from build123d import *

# Parameters (mm, degrees)
SKETCH1_R           = 12.5
BOSS_EXTRUDE1_DEPTH = 25
SKETCH2_R           = 5
CUT_EXTRUDE1_DEPTH  = 20
SKETCH4_R           = 2
CUT_EXTRUDE2_DEPTH  = 20
SKETCH5_R           = 28.5
SKETCH5_R_2         = 2.6
BOSS_EXTRUDE2_DEPTH = 6
SKETCH6_R           = 9
BOSS_EXTRUDE3_DEPTH = 80.52
SKETCH7_R           = 8.5
BOSS_EXTRUDE4_DEPTH = 20.5
SKETCH8_R           = 10.9
BOSS_EXTRUDE5_DEPTH = 18


with BuildPart() as part:
    # Sketch1 → Boss-Extrude1 (new body)
    with BuildSketch(Plane.XY):
        Circle(SKETCH1_R)
    extrude(amount=BOSS_EXTRUDE1_DEPTH)

    # Sketch2 → Cut-Extrude1 (cut)
    with BuildSketch(Plane(origin=(0, 0, 0), x_dir=(-1, 0, 0), z_dir=(0, 0, -1))):
        Circle(SKETCH2_R)
    extrude(amount=-CUT_EXTRUDE1_DEPTH, mode=Mode.SUBTRACT)

    # Sketch4 → Cut-Extrude2 (cut)
    with BuildSketch(Plane(origin=(0, 0, 0), x_dir=(1, 0, 0), z_dir=(0, 1, 0))):
        with Locations(Location((0, -8, 0), (0, 0, 270))):
            Circle(SKETCH4_R)
    extrude(amount=-CUT_EXTRUDE2_DEPTH, mode=Mode.SUBTRACT)

    # Sketch5 → Boss-Extrude2 (add)
    with BuildSketch(Plane.XY.offset(25)):
        Circle(SKETCH5_R)
        with Locations((0, 23.75)):
            Circle(SKETCH5_R_2, mode=Mode.SUBTRACT)
        with Locations((20.56810334, 11.875)):
            Circle(SKETCH5_R_2, mode=Mode.SUBTRACT)
        with Locations((20.56810334, -11.875)):
            Circle(SKETCH5_R_2, mode=Mode.SUBTRACT)
        with Locations((0, -23.75)):
            Circle(SKETCH5_R_2, mode=Mode.SUBTRACT)
        with Locations((-20.56810334, -11.875)):
            Circle(SKETCH5_R_2, mode=Mode.SUBTRACT)
        with Locations((-20.56810334, 11.875)):
            Circle(SKETCH5_R_2, mode=Mode.SUBTRACT)
    extrude(amount=BOSS_EXTRUDE2_DEPTH)

    # Sketch6 → Boss-Extrude3 (add)
    with BuildSketch(Plane.XY.offset(31)):
        Circle(SKETCH6_R)
    extrude(amount=BOSS_EXTRUDE3_DEPTH)

    # Sketch7 → Boss-Extrude4 (add)
    with BuildSketch(Plane.XY.offset(111.52)):
        Circle(SKETCH7_R)
    extrude(amount=BOSS_EXTRUDE4_DEPTH)

    # Sketch8 → Boss-Extrude5 (add)
    with BuildSketch(Plane.XY.offset(31)):
        Circle(SKETCH8_R)
    extrude(amount=BOSS_EXTRUDE5_DEPTH)


solid = part.part
CAD build for the part. Positions are in the model's coordinates, mm. A direction names the side the tool comes from. Give positions to 0.01 mm unless a question says otherwise; leave off trailing zeros. Order: outer loops, then holes, each group sorted by start corner. A loop starts at its lowest first (then second) coordinate and runs counter-clockwise, first axis right, second up. Notation, with made-up numbers: (-4.5, 34) -> (18.5, 34) arc R24 ccw to (18.5, 45) -> close; hole circle Ø8 at (66, 36.5). An arc over 180 degrees is marked (long way). Return JSON: item names as keys, results as strings.
Q1. Saw through at D-D (z = 15.5). Write the cut outline in (x, y), then the cut area to 3 significant figures.
Working result:
{"outline": "circle Ø25 at (0, 0); hole circle Ø10 at (0, 0)", "area": "412 mm²"}
Q2. Drill centre lines: line 1 (Y direction, x = 0, z = 28); line 2 (Z direction, x = 0, y = -6.25); line 3 (Y direction, x = 18.5, z = 27). Where is each one in solid material? Low to high.
Working result:
{"line 1": "-28.5 to -26.35, -21.15 to 21.15, 26.35 to 28.5", "line 2": "0 to 6, 10 to 132.02", "line 3": "-21.68 to -13.45, -10.3 to 10.3, 13.45 to 21.68"}
Q3. Mould opens along X. For faces 1 (the face through (21.77, 9.57, 27.96)), 2 (the face through (-1.172, 8.923, 79.822)), 3 (the face through (-19.368, 9.568, 27.958)), 4 (the face through (-0.2, -5.4, 0)) say: pulls with the +X half, pulls with the -X half, needs draft (parallel to the pull), parting line crosses it, or undercut.
Working result:
{"face 1": "undercut", "face 2": "parting line crosses it", "face 3": "undercut", "face 4": "needs draft"}
Q4. Saw through at B-B (x = 20). Write the cut outline in (y, z), then the cut area to 3 significant figures.
Working result:
{"outline": "(-20.3, 25) -> (-14.41, 25) -> (-14.41, 31) -> (-20.3, 31) -> close; (-9.34, 25) -> (9.34, 25) -> (9.34, 31) -> (-9.34, 31) -> close; (14.41, 25) -> (20.3, 25) -> (20.3, 31) -> (14.41, 31) -> close", "area": "183 mm²"}
Q5. Which spindle directions (+Z, -Z, +X, -X, +Y, -Y) get a long thin tool onto all of the face, cutting with end or side? Do faces 5 (the face through (2, 9, 49)), 6 (the face through (0, 0, 132.02)), 7 (the face through (-0.338, 26.328, 27.958)), 8 (the face through (-0.766, -8.488, 9.847)), 9 (the face through (11.923, 3.755, 12.325)). Say none if no direction does.
Working result:
{"face 5": "+Z", "face 6": "+Z, +X, -X, +Y, -Y", "face 7": "+Z, -Z", "face 8": "-Y", "face 9": "-Z"}
Q6. Saw through at A-A (y = -23.75). Write the cut outline in (x, z).
Working result:
{"outline": "(-15.75, 25) -> (-2.6, 25) -> (-2.6, 31) -> (-15.75, 31) -> close; (2.6, 25) -> (15.75, 25) -> (15.75, 31) -> (2.6, 31) -> close"}
Q7. Flat gauge pins, fed straight in: pin 1 (1 mm diameter, centred on x = 9.5, y = -18.5, fed in from -Z); pin 2 (12 mm diameter, centred on y = 1, z = 103.5, fed in from -X); pin 3 (6 mm diameter, centred on x = 0, y = -23.75, fed in from +Z). Where does each tip first touch, or does it go through?
Working result:
{"pin 1": "z = 25", "pin 2": "x = -9", "pin 3": "z = 31"}
Q8. Saw through at C-C (y = 0). Write the cut outline in (x, z).
Working result:
{"outline": "(-28.5, 25) -> (-12.5, 25) -> (-12.5, 0) -> (-5, 0) -> (-5, 20) -> (5, 20) -> (5, 0) -> (12.5, 0) -> (12.5, 25) -> (28.5, 25) -> (28.5, 31) -> (10.9, 31) -> (10.9, 49) -> (9, 49) -> (9, 111.52) -> (8.5, 111.52) -> (8.5, 132.02) -> (-8.5, 132.02) -> (-8.5, 111.52) -> (-9, 111.52) -> (-9, 49) -> (-10.9, 49) -> (-10.9, 31) -> (-28.5, 31) -> close"}
